```python
from build123d import *

# Parameters (mm, degrees)
BOSS_EXTRUDE1_DEPTH     = 4.7625
CUT_EXTRUDE1_DEPTH      = 26.250733281
CUT_EXTRUDE1_DEPTH_BACK = 26.250733281
SKETCH2_R               = 2.1828125
CUT_EXTRUDE2_DEPTH      = 29.794641971
CUT_EXTRUDE2_DEPTH_BACK = 29.794641971
SKETCH3_R               = 2.38125
FILLET1_R               = 4.7625
FILLET2_R               = 1.5875
CHAMFER1_SIZE           = 0.396875


with BuildPart() as part:
    # Sketch1 → Boss-Extrude1 (new, symmetric)
    with BuildSketch(Plane(origin=(0, 0, 0), x_dir=(1, 0, 0), z_dir=(0, 1, 0))):
        Polygon((0, 0), (19.05, 0), (19.05, 9.525), (6.35, 9.525), (6.35, 25.4), (0, 25.4), align=None)
    extrude(amount=BOSS_EXTRUDE1_DEPTH, both=True)

    # Sketch2 → Cut-Extrude1 (cut, two sides: drawn at the far end of the back side and taken through both)
    with BuildSketch(Plane(origin=(0, 0, -9.525), x_dir=(-1, 0, 0), z_dir=(0, 0, -1)).offset(-CUT_EXTRUDE1_DEPTH_BACK)):
        with Locations((-14.2875, 0)):
            Circle(SKETCH2_R)
    extrude(amount=CUT_EXTRUDE1_DEPTH + CUT_EXTRUDE1_DEPTH_BACK, mode=Mode.SUBTRACT)

    # Sketch3 → Cut-Extrude2 (cut, two sides: drawn at the far end of the back side and taken through both)
    with BuildSketch(Plane(origin=(6.35, 0, 0), x_dir=(0, 0, -1), z_dir=(1, 0, 0)).offset(-CUT_EXTRUDE2_DEPTH_BACK)):
        with Locations((20.6375, 0)):
            Circle(SKETCH3_R)
    extrude(amount=CUT_EXTRUDE2_DEPTH + CUT_EXTRUDE2_DEPTH_BACK, mode=Mode.SUBTRACT)

    # Fillet1
    fillet1_edges = [part.edges().sort_by_distance(p)[0] for p in [
        (0, 0, 0),
        (3.175, -4.7625, -25.4),
        (3.175, 4.7625, -25.4),
        (19.05, -4.7625, -4.7625),
        (19.05, 4.7625, -4.7625),
    ]]
    fillet(fillet1_edges, radius=FILLET1_R - 0.0001)  # a hair under: the kernel refuses the full size

    # Fillet2
    fillet2_edges = [part.edges().sort_by_distance(p)[0] for p in [
        (6.35, 0, -9.525),
    ]]
    fillet(fillet2_edges, radius=FILLET2_R)

    # Chamfer1
    chamfer1_edges = [part.edges().sort_by_distance(p)[0] for p in [
        (16.4703125, 0, 0),
        (16.4703125, 0, -9.525),
        (0, 0, -18.25625),
        (6.35, 0, -18.25625),
        (9.525, -4.7625, 0),
        (9.525, 4.7625, 0),
        (17.655125335, 3.367625335, 0),
        (17.655125335, -3.367625335, 0),
        (0, -4.7625, -12.7),
        (11.11255, -4.7625, -9.525),
        (1.394874665, -4.7625, -1.394874665),
        (0, 4.7625, -12.7),
        (0, 3.367625335, -24.005125335),
        (0, -3.367625335, -24.005125335),
        (11.11255, 4.7625, -9.525),
        (1.394874665, 4.7625, -1.394874665),
        (6.35, 3.367625335, -24.005125335),
        (6.35, -3.367625335, -24.005125335),
        (17.655125335, 3.367625335, -9.525),
        (17.655125335, -3.367625335, -9.525),
        (6.35, -4.7625, -15.87505),
        (6.35, 4.7625, -15.87505),
        (6.814967985, -4.7625, -9.989967985),
        (6.814967985, 4.7625, -9.989967985),
    ]]
    chamfer(chamfer1_edges, length=CHAMFER1_SIZE)


solid = part.part
```
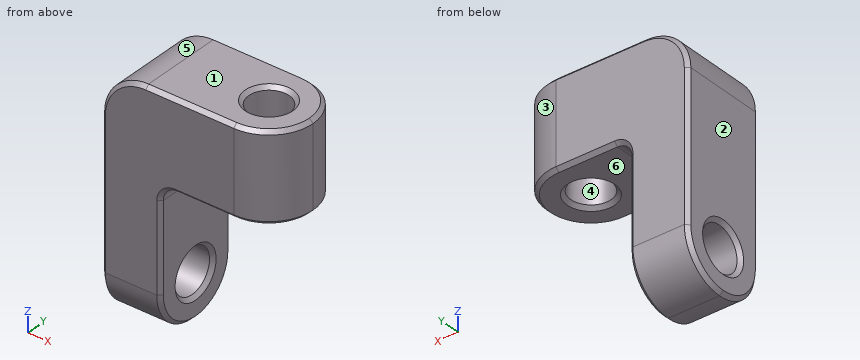
Work out the finished part from the listing and answer in its coordinate system (mm). Face numbers are marked on the shaded views. A direction names the side the tool comes from. Coordinates: 2 decimals unless noted, no trailing zeros. Loops run counter-clockwise (first coordinate to the right, second up) from the corner with the lowest first, then second, coordinate; pieces in that order, holes last. Notation, with made-up numbers: (83.5, 66) - (93.5, 66) arc R27 cw to (93.5, 102) - close; hole circle Ø4 at (37.25, -6). An arc over 180 degrees is marked (long way). Use a Markdown table: item, result.
Item 1: Find section A-A, the plane z = -12.5. Determine the outline of the cut face in (x, y), and give its area (3 significant figures).
Evaluation:
| item | result |
|---|---|
| outline | (0, -4.37) - (0.4, -4.76) - (5.95, -4.76) - (6.35, -4.37) - (6.35, 4.37) - (5.95, 4.76) - (0.4, 4.76) - (0, 4.37) - close |
| area | 60.2 mm2 |
Item 2: For the marked faces 5 and 6, determine the directions among +Z, -Z, +X, -X, +Y, -Y from which every point of the face is accessible in a straight line to the end or side of a thin tool.
Evaluation:
| item | result |
|---|---|
| face 5 | +Z, -X, +Y, -Y |
| face 6 | -Z, +X, +Y, -Y |
Item 3: Given pin 1 Ø4.5 at (y, z) = (1.5, -15.5) entering from +X; pin 2 Ø5 at (x, y) = (4.5, 3.5) entering from -Z, each flat-ended and moving along its own axis, determine where each tip first touches the part or whether it passes through.
Evaluation:
| item | result |
|---|---|
| pin 1 | stops at x = 6.35 |
| pin 2 | stops at z = -25.29 |
Item 4: Find section B-B, the plane x = 10. Determine the outline of the cut face in (y, z) (1 decimal), and give its area (3 significant figures).
Evaluation:
| item | result |
|---|---|
| outline | (-4.8, -9.1) - (-4.4, -9.5) - (4.4, -9.5) - (4.8, -9.1) - (4.8, -0.4) - (4.4, 0) - (-4.4, 0) - (-4.8, -0.4) - close |
| area | 90.4 mm2 |
Item 5: Consider probe 1 along X at (y, z) = (2, -12.75); probe 2 along Y at (x, z) = (12.75, -4.25); probe 3 along Z at (x, y) = (2.95, 0). Determine where each line is inside the solid, lowest interval first. Write a range as from..to.
Evaluation:
| item | result |
|---|---|
| probe 1 | x = 0..6.35 |
| probe 2 | y = -4.76..-1.55, 1.55..4.76 |
| probe 3 | z = -25.4..-23.02, -18.26..-0.36 |
Item 6: Find section C-C, the plane y = -1.5. State how many separate pieces and enclosed holes the cut face has, and give its area (3 significant figures).
Evaluation:
| item | result |
|---|---|
| separate pieces | 3 |
| enclosed holes | 0 |
| area | 219 mm2 |
Item 7: The mould has two halves that part along X. Classify the marked faces 1, 2, 3 and 4: +X half, -X half, draft (parallel to the pull), parting line (faces both ways), or undercut.
Evaluation:
| item | result |
|---|---|
| face 1 | draft |
| face 2 | -X half |
| face 3 | +X half |
| face 4 | undercut |
